```python
from build123d import *

# Parameters (mm, degrees)
BOSS_EXTRUDE1_DEPTH = 1.5
SKETCH2_W           = 10.6
SKETCH2_H           = 11.5
BOSS_EXTRUDE2_DEPTH = 4
BOSS_EXTRUDE4_DEPTH = 6.07
SKETCH5_W           = 1.5
SKETCH5_H           = 2.5
BOSS_EXTRUDE5_DEPTH = 4.5
SKETCH6_W           = 0.5
SKETCH6_H           = 2.5
CUT_EXTRUDE1_DEPTH  = 16.632418239
SKETCH7_W           = 0.5
SKETCH7_H           = 2.5
SKETCH7_H_2         = 1
CUT_EXTRUDE3_DEPTH  = 4
SKETCH8_W           = 8
SKETCH8_H           = 6.07
CUT_EXTRUDE4_DEPTH  = 15.121260567
SKETCH10_R          = 1.75
CUT_EXTRUDE5_DEPTH  = 4.75
SKETCH12_W          = 2.7
SKETCH12_H          = 4
BOSS_EXTRUDE6_DEPTH = 0.75
SKETCH13_W          = 2.7
SKETCH13_H          = 4
BOSS_EXTRUDE7_DEPTH = 0.75
CUT_EXTRUDE6_DEPTH  = 17.633099531
CUT_EXTRUDE7_DEPTH  = 12.636580254
SKETCH17_W          = 9.1
SKETCH17_H          = 2.975518652
CUT_EXTRUDE8_DEPTH  = 0.5
FILLET2_R           = 1
SKETCH18_W          = 8.152515879
SKETCH18_H          = 2.332912786
CUT_EXTRUDE9_DEPTH  = 4
SKETCH19_W          = 1.745
SKETCH19_H          = 0.376419973
SKETCH19_W_2        = 1.75
CUT_EXTRUDE10_DEPTH = 4
SKETCH20_W          = 1.5
SKETCH20_H          = 4
CUT_EXTRUDE11_DEPTH = 4


with BuildPart() as part:
    # Sketch1 → Boss-Extrude1 (new body)
    with BuildSketch(Plane(origin=(0, 0, 0), x_dir=(1, 0, 0), z_dir=(0, 1, 0))):
        with BuildLine():
            Line((-6, -7.1), (6, -7.1))
            ThreePointArc((6, -7.1), (6.707106781, -6.807106781), (7, -6.1))
            Line((7, -6.1), (7, 6.1))
            ThreePointArc((7, 6.1), (6.707106781, 6.807106781), (6, 7.1))
            Line((6, 7.1), (-6, 7.1))
            ThreePointArc((-6, 7.1), (-6.707106781, 6.807106781), (-7, 6.1))
            Line((-7, 6.1), (-7, -6.1))
            ThreePointArc((-7, -6.1), (-6.707106781, -6.807106781), (-6, -7.1))
        make_face()
    extrude(amount=BOSS_EXTRUDE1_DEPTH)

    # Sketch2 → Boss-Extrude2 (add)
    with BuildSketch(Plane(origin=(0, 1.5, 0), x_dir=(1, 0, 0), z_dir=(0, 1, 0))):
        with Locations((0, 1.35)):
            Rectangle(SKETCH2_W, SKETCH2_H)
    extrude(amount=BOSS_EXTRUDE2_DEPTH)

    # Sketch4 → Boss-Extrude4 (add)
    with BuildSketch(Plane.XY.offset(3)):
        Polygon((-5.3, 5.5), (-7, 1.5), (-5.3, 1.5), align=None)
        Polygon((5.3, 5.5), (7, 1.5), (5.3, 1.5), align=None)
    extrude(amount=-BOSS_EXTRUDE4_DEPTH)

    # Sketch5 → Boss-Extrude5 (add)
    with BuildSketch(Plane.XZ):
        with Locations((-6.25, 4.5)):
            Rectangle(SKETCH5_W, SKETCH5_H)
        with Locations((6.25, 4.5)):
            Rectangle(SKETCH5_W, SKETCH5_H)
        with Locations((6.25, -4.5)):
            Rectangle(SKETCH5_W, SKETCH5_H)
        with Locations((-6.25, -4.5)):
            Rectangle(SKETCH5_W, SKETCH5_H)
    extrude(amount=BOSS_EXTRUDE5_DEPTH)

    # Sketch6 → Cut-Extrude1 (cut, through all)
    with BuildSketch(Plane.XY.offset(5.75)):
        with Locations((-5.75, -1.25)):
            Rectangle(SKETCH6_W, SKETCH6_H)
        Polygon((-7, -4.5), (-7, -3), (-6.5, -4.5), align=None)
        Polygon((-5.5, -3), (-6, -4.5), (-5.5, -4.5), align=None)
        with Locations((5.75, -1.25)):
            Rectangle(SKETCH6_W, SKETCH6_H)
        Polygon((5.5, -3), (6, -4.5), (5.5, -4.5), align=None)
        Polygon((7, -4.5), (7, -3), (6.5, -4.5), align=None)
    extrude(amount=-CUT_EXTRUDE1_DEPTH, mode=Mode.SUBTRACT)

    # Sketch7 → Cut-Extrude3 (cut)
    with BuildSketch(Plane(origin=(0, 1.5, 0), x_dir=(1, 0, 0), z_dir=(0, 1, 0))):
        with Locations((5.75, -4.5)):
            Rectangle(SKETCH7_W, SKETCH7_H)
        with Locations((6.25, -4.5)):
            Rectangle(SKETCH7_W, SKETCH7_H_2)
        with Locations((-6.25, -4.5)):
            Rectangle(SKETCH7_W, SKETCH7_H_2)
        with Locations((-5.75, -4.5)):
            Rectangle(SKETCH7_W, SKETCH7_H)
        with Locations((5.75, 4.5)):
            Rectangle(SKETCH7_W, SKETCH7_H)
        with Locations((6.25, 4.5)):
            Rectangle(SKETCH7_W, SKETCH7_H_2)
        with Locations((-5.75, 4.5)):
            Rectangle(SKETCH7_W, SKETCH7_H)
        with Locations((-6.25, 4.5)):
            Rectangle(SKETCH7_W, SKETCH7_H_2)
    extrude(amount=-CUT_EXTRUDE3_DEPTH, mode=Mode.SUBTRACT)

    # Sketch8 → Cut-Extrude4 (cut, through all)
    with BuildSketch(Plane(origin=(0, 5.5, 0), x_dir=(1, 0, 0), z_dir=(0, 1, 0))):
        with Locations((0, 0.035)):
            Rectangle(SKETCH8_W, SKETCH8_H)
    extrude(amount=-CUT_EXTRUDE4_DEPTH, mode=Mode.SUBTRACT)

    # Sketch10 → Cut-Extrude5 (cut)
    with BuildSketch(Plane(origin=(0, 5.5, 0), x_dir=(1, 0, 0), z_dir=(0, 1, 0))):
        with Locations((0, -5.5)):
            Circle(SKETCH10_R)
    extrude(amount=-CUT_EXTRUDE5_DEPTH, mode=Mode.SUBTRACT)

    # Sketch12 → Boss-Extrude6 (add)
    with BuildSketch(Plane.ZY.offset(5.3)):
        with Locations((5.75, 3.5)):
            Rectangle(SKETCH12_W, SKETCH12_H)
    extrude(amount=-BOSS_EXTRUDE6_DEPTH)

    # Sketch13 → Boss-Extrude7 (add)
    with BuildSketch(Plane(origin=(5.3, 0, 0), x_dir=(0, 0, -1), z_dir=(1, 0, 0))):
        with Locations((-5.75, 3.5)):
            Rectangle(SKETCH13_W, SKETCH13_H)
    extrude(amount=-BOSS_EXTRUDE7_DEPTH)

    # Sketch15 → Cut-Extrude6 (cut, through all)
    with BuildSketch(Plane(origin=(7, 0, 0), x_dir=(0, 0, -1), z_dir=(1, 0, 0))):
        Polygon((-4.4, 5.5), (-7.1, 0), (-7.1, 5.5), align=None)
        Polygon((7.1, 0), (6.1, 5.5), (7.1, 5.5), align=None)
    extrude(amount=-CUT_EXTRUDE6_DEPTH, mode=Mode.SUBTRACT)

    # Sketch16 → Cut-Extrude7 (cut, through all)
    with BuildSketch(Plane(origin=(0, 1.5, 0), x_dir=(1, 0, 0), z_dir=(0, 1, 0))):
        with BuildLine():
            Line((-3.586359169, -5.147740482), (3.606419083, -5.147740482))
            ThreePointArc((3.606419083, -5.147740482), (3.856419083, -5.397740482), (3.606419083, -5.647740482))
            Line((3.606419083, -5.647740482), (-3.586359169, -5.647740482))
            ThreePointArc((-3.586359169, -5.647740482), (-3.836359169, -5.397740482), (-3.586359169, -5.147740482))
        make_face()
    extrude(amount=-CUT_EXTRUDE7_DEPTH, mode=Mode.SUBTRACT)

    # Sketch17 → Cut-Extrude8 (cut)
    with BuildSketch(Plane(origin=(0, 1.5, 0), x_dir=(1, 0, 0), z_dir=(0, 1, 0))):
        with Locations((0, -5.887759326)):
            Rectangle(SKETCH17_W, SKETCH17_H)
    extrude(amount=-CUT_EXTRUDE8_DEPTH, mode=Mode.SUBTRACT)

    # Fillet2
    fillet2_edges = [part.edges().sort_by_distance(p)[0] for p in [
        (0, 5.5, -6.1),
    ]]
    fillet(fillet2_edges, radius=FILLET2_R)

    # Sketch18 → Cut-Extrude9 (cut)
    with BuildSketch(Plane.XZ):
        with Locations((0.100583502, -4.612876366)):
            Rectangle(SKETCH18_W, SKETCH18_H)
    extrude(amount=-CUT_EXTRUDE9_DEPTH, mode=Mode.SUBTRACT)

    # Sketch19 → Cut-Extrude10 (cut)
    with BuildSketch(Plane.XZ):
        with Locations((3.1275, -3.258209987)):
            Rectangle(SKETCH19_W, SKETCH19_H)
        with Locations((-3.100674438, -3.258209987)):
            Rectangle(SKETCH19_W_2, SKETCH19_H)
    extrude(amount=-CUT_EXTRUDE10_DEPTH, mode=Mode.SUBTRACT)

    # Sketch20 → Cut-Extrude11 (cut)
    with BuildSketch(Plane.XZ):
        with Locations((4.75, -0.051196063)):
            Rectangle(SKETCH20_W, SKETCH20_H)
        with Locations((-4.75, -0.051196063)):
            Rectangle(SKETCH20_W, SKETCH20_H)
    extrude(amount=-CUT_EXTRUDE11_DEPTH, mode=Mode.SUBTRACT)


solid = part.part
```
Can you work these out from the model? Positions are in its coordinate system, mm. A direction names the side the tool comes from. Round coordinates to 2 decimals unless told otherwise and drop trailing zeros. Loops run counter-clockwise (first coordinate to the right, second up) from the corner with the lowest first, then second, coordinate; pieces in that order, holes last.
Item 1: Will these pins go through, and if not, where does the flat tip stop? pin 1 Ø0.6 at (x, y) = (-5.5, 0.5) entering from +Z; pin 2 Ø0.5 at (x, z) = (-6, -5) entering from +Y; pin 3 Ø1.5 at (y, z) = (-2, 0) entering from +X; pin 4 Ø0.8 at (y, z) = (2, -4.5) entering from +X.
Item 2: Suppose I cut it at D-D, the plane x = -5. Write out the boundary of the cut face in (y, z), then the cut area to 3 significant figures.
Item 3: Suppose I cut it at A-A, the plane x = -2.5. Write out the boundary of the cut face in (y, z).
Item 4: If we mould it in two halves opening along Z, with no side actions, what happens to faces 6 (the flat face through (4.177, 2, -5)), 7 (the flat face through (5.5, 1, -4)), 8 (the flat face through (-0.483, 0.522, 6.844)), 9 (the flat face through (-5.3, 3, -5))? For each: +Z half, -Z half, draft (parallel to the pull), parting line (faces both ways), or undercut.
Item 5: Suppose I cut it at B-B, the plane y = -1. State how many separate pieces and enclosed holes the cut face has, then the cut area to 3 significant figures.
Item 6: Please list where these lines run through material, in increasing order: L1, parallel to X at y = 3, z = 4.5; L2, parallel to X at y = -0.25, z = -5.25; L3, parallel to Z at x = -0.75, y = 1.75.
Item 7: Which directions (+Z, -Z, +X, -X, +Y, -Y) give clear straight access to the entire face, cutting with the end or side of a thin tool? Please do faces 1 (the flat face through (6.4, -2.2, -3.25)), 2 (the flat face through (-5.746, -3.74, -4.482)), 3 (the flat face through (-5.3, 3, 4)), 4 (the flat face through (-5, 2, 1.949)), 5 (the flat face through (0.1, 0.5, 5.648)).
Item 8: Suppose I cut it at C-C, the plane z = 1. Write out the boundary of the cut face in (x, y).
Reported:
1. pin 1: stops at z = 7
1. pin 2: stops at y = 1.5
1. pin 3: passes through
1. pin 4: stops at x = 5.3
2. outline: (0, -7.1) - (4.68, -6.25) arc R1 ccw to (5.5, -5.27) - (5.5, 4.4) - (0, 7.1) - (0, 1.95) - (4, 1.95) - (4, -2.05) - (0, -2.05) - close
2. area: 51.8 mm2
3. outline: (0, -7.1) - (4.68, -6.25) arc R1 ccw to (5.5, -5.27) - (5.5, -3.07) - (4, -3.07) - (4, -5.78) - (0, -5.78) - close; (0, 3) - (5.5, 3) - (5.5, 4.4) - (1, 4.4) - (1, 5.15) - (0, 5.15) - close; (0, 5.65) - (1, 5.65) - (1, 6.61) - (0, 7.1) - close
4. face 6: undercut
4. face 7: undercut
4. face 8: +Z half
4. face 9: draft
5. separate pieces: 4
5. enclosed holes: 0
5. area: 8.00 mm2
6. L1: x = -5.3 to -4.55, 4.55 to 5.3
6. L2: x = -7 to -6, 6 to 7
6. L3: z = -6.78 to -5.78, -3.45 to -3.07, 3 to 3.92
7. face 1: +X, -X, -Y
7. face 2: +Z, -Z, -Y
7. face 3: +Z, -X, +Y
7. face 4: -Y
7. face 5: +Y, -Y
8. outline: (-7, 0) - (-5.5, 0) - (-5.5, 4) - (-4, 4) - (-4, 5.5) - (-5.3, 5.5) - (-7, 1.5) - close; (4, 4) - (5.5, 4) - (5.5, 0) - (7, 0) - (7, 1.5) - (5.3, 5.5) - (4, 5.5) - close
